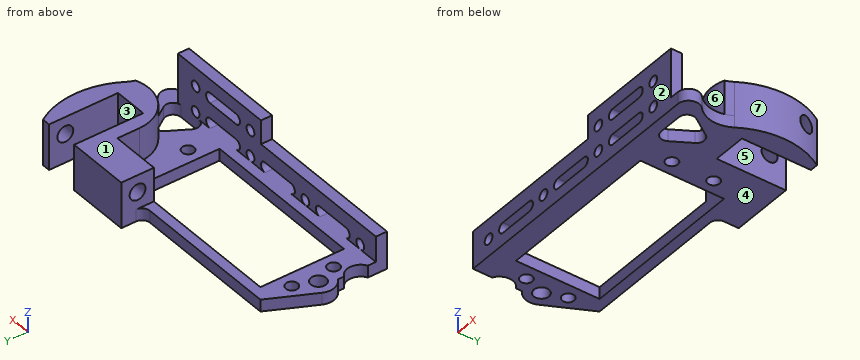
from build123d import *

# Parameters (mm, degrees)
SKETCH1_R           = 1.5
SKETCH1_R_2         = 1.9
SKETCH1_W           = 41.5
SKETCH1_H           = 21
BOSS_EXTRUDE1_DEPTH = 3
BOSS_EXTRUDE2_DEPTH = 8.5
BOSS_EXTRUDE3_DEPTH = 12.4
SKETCH4_R           = 1.3
CUT_EXTRUDE1_DEPTH  = 12.4
SKETCH5_W           = 38.3
SKETCH5_H           = 6
CUT_EXTRUDE2_DEPTH  = 12.4
SKETCH6_R           = 2
CUT_EXTRUDE3_DEPTH  = 42.4


with BuildPart() as part:
    # Sketch1 → Boss-Extrude1 (new body)
    with BuildSketch(Plane.XY):
        with BuildLine():
            Line((-3.321392505, 23.5), (33.5, 23.5))
            ThreePointArc((33.5, 23.5), (34.914213562, 24.085786438), (35.5, 25.5))
            Line((35.5, 25.5), (35.5, 29.2))
            Line((35.5, 29.2), (51.2, 29.2))
            Line((51.2, 29.2), (51.2, 11.85))
            Line((51.2, 11.85), (59.6, 11.85))
            Line((59.6, 11.85), (59.6, 29.2))
            Line((59.6, 29.2), (61.598774259, 29.2))
            ThreePointArc((61.598774259, 29.2), (64.6, 18.815792472), (61.598774259, 8.431584945))
            ThreePointArc((61.598774259, 8.431584945), (60.564280065, 3.6748318), (62.825022394, -0.636307591))
            ThreePointArc((62.825022394, -0.636307591), (63.518866569, -3.587010054), (61.018120639, -5.3))
            Line((61.018120639, -5.3), (-7.3, -5.3))
            Line((-7.3, -5.3), (-7.3, -0.5))
            ThreePointArc((-7.3, -0.5), (-5.5, 2.5), (-7.3, 5.5))
            Line((-7.3, 5.5), (-7.3, 7.067398479))
            ThreePointArc((-7.3, 7.067398479), (-9.16671437, 9.322502878), (-8.93851269, 12.241071429))
            Line((-8.93851269, 12.241071429), (-3.321392505, 23.5))
        make_face()
        with Locations((-3.5, 15.75)):
            Circle(SKETCH1_R, mode=Mode.SUBTRACT)
        with Locations((-5.448717527, 10.5)):
            Circle(SKETCH1_R_2, mode=Mode.SUBTRACT)
        with Locations((-3.5, 5.25)):
            Circle(SKETCH1_R, mode=Mode.SUBTRACT)
        with Locations((45, 5.25)):
            Circle(SKETCH1_R, mode=Mode.SUBTRACT)
        with Locations((45, 15.75)):
            Circle(SKETCH1_R, mode=Mode.SUBTRACT)
        with Locations((20.75, 10.5)):
            Rectangle(SKETCH1_W, SKETCH1_H, mode=Mode.SUBTRACT)
        with BuildLine():
            Line((49.961498231, 0.517681209), (52.768212791, 5.266104179))
            ThreePointArc((52.768212791, 5.266104179), (54.433574671, 6.247628711), (56.151588007, 5.361484945))
            Line((56.151588007, 5.361484945), (59.33232839, 0.613061975))
            ThreePointArc((59.33232839, 0.613061975), (59.435061822, -1.441773872), (57.670674684, -2.5))
            Line((57.670674684, -2.5), (51.683219741, -2.5))
            ThreePointArc((51.683219741, -2.5), (49.946072306, -1.491119968), (49.961498231, 0.517681209))
        make_face(mode=Mode.SUBTRACT)
    extrude(amount=BOSS_EXTRUDE1_DEPTH)

    # Sketch2 → Boss-Extrude2 (add)
    with BuildSketch(Plane.XY.offset(3)):
        with BuildLine():
            Line((61.598774259, 29.2), (59.6, 29.2))
            Line((59.6, 29.2), (59.6, 11.85))
            Line((59.6, 11.85), (51.2, 11.85))
            Line((51.2, 11.85), (51.2, 29.2))
            Line((51.2, 29.2), (35.5, 29.2))
            Line((35.5, 29.2), (35.5, 21))
            Line((35.5, 21), (47.7, 21))
            Line((47.7, 21), (47.7, 15.472440326))
            ThreePointArc((47.7, 15.472440326), (51.882998061, 7.567370729), (60.771830096, 6.579310435))
            ThreePointArc((60.771830096, 6.579310435), (61.119060066, 7.535021345), (61.598774259, 8.431584945))
            ThreePointArc((61.598774259, 8.431584945), (64.6, 18.815792472), (61.598774259, 29.2))
        make_face()
    extrude(amount=BOSS_EXTRUDE2_DEPTH)

    # Sketch3 → Boss-Extrude3 (add)
    with BuildSketch(Plane.XY.offset(3)):
        Polygon((46.39680607, -5.3), (-7.3, -5.3), (-7.3, -2.5), (58.7, -2.5), (58.7, -5.3), align=None)
    extrude(amount=BOSS_EXTRUDE3_DEPTH)

    # Sketch4 → Cut-Extrude1 (cut)
    with BuildSketch(Plane(origin=(0, -2.5, 0), x_dir=(1, 0, 0), z_dir=(0, 1, 0))):
        with Locations((52.8, -4.3)):
            Circle(SKETCH4_R)
        with Locations((34.5, -4.3)):
            Circle(SKETCH4_R)
        with Locations((52.8, -10.7)):
            Circle(SKETCH4_R)
        with Locations((34.5, -10.7)):
            Circle(SKETCH4_R)
        with Locations((16.2, -10.7)):
            Circle(SKETCH4_R)
        with Locations((-2.1, -10.7)):
            Circle(SKETCH4_R)
        with Locations((16.2, -4.3)):
            Circle(SKETCH4_R)
        with Locations((-2.1, -4.3)):
            Circle(SKETCH4_R)
        with BuildLine():
            Line((48, -5.6), (39.3, -5.6))
            ThreePointArc((39.3, -5.6), (38, -4.3), (39.3, -3))
            Line((39.3, -3), (48, -3))
            ThreePointArc((48, -3), (49.3, -4.3), (48, -5.6))
        make_face()
        with BuildLine():
            Line((48, -12), (39.3, -12))
            ThreePointArc((39.3, -12), (38, -10.7), (39.3, -9.4))
            Line((39.3, -9.4), (48, -9.4))
            ThreePointArc((48, -9.4), (49.3, -10.7), (48, -12))
        make_face()
        with BuildLine():
            Line((29.7, -12), (21, -12))
            ThreePointArc((21, -12), (19.7, -10.7), (21, -9.4))
            Line((21, -9.4), (29.7, -9.4))
            ThreePointArc((29.7, -9.4), (31, -10.7), (29.7, -12))
        make_face()
        with BuildLine():
            Line((11.4, -12), (2.7, -12))
            ThreePointArc((2.7, -12), (1.4, -10.7), (2.7, -9.4))
            Line((2.7, -9.4), (11.4, -9.4))
            ThreePointArc((11.4, -9.4), (12.7, -10.7), (11.4, -12))
        make_face()
        with BuildLine():
            Line((29.7, -5.6), (21, -5.6))
            ThreePointArc((21, -5.6), (19.7, -4.3), (21, -3))
            Line((21, -3), (29.7, -3))
            ThreePointArc((29.7, -3), (31, -4.3), (29.7, -5.6))
        make_face()
        with BuildLine():
            Line((11.4, -5.6), (2.7, -5.6))
            ThreePointArc((2.7, -5.6), (1.4, -4.3), (2.7, -3))
            Line((2.7, -3), (11.4, -3))
            ThreePointArc((11.4, -3), (12.7, -4.3), (11.4, -5.6))
        make_face()
    extrude(amount=-CUT_EXTRUDE1_DEPTH, mode=Mode.SUBTRACT)

    # Sketch5 → Cut-Extrude2 (cut)
    with BuildSketch(Plane(origin=(0, -2.5, 0), x_dir=(1, 0, 0), z_dir=(0, 1, 0))):
        with Locations((11.85, -12.4)):
            Rectangle(SKETCH5_W, SKETCH5_H)
    extrude(amount=-CUT_EXTRUDE2_DEPTH, mode=Mode.SUBTRACT)

    # Sketch6 → Cut-Extrude3 (cut)
    with BuildSketch(Plane.ZY.offset(-35.5)):
        with Locations((7.25, 25.1)):
            Circle(SKETCH6_R)
    extrude(amount=-CUT_EXTRUDE3_DEPTH, mode=Mode.SUBTRACT)


solid = part.part
Design review of the part built by this model. Coordinates are the model's own, in mm. Face numbers are marked on the shaded views. A direction names the side the tool comes from. Coordinates: 2 decimals unless noted, no trailing zeros. Write each loop counter-clockwise with the first axis right and the second up, starting at its lowest first coordinate (ties: lowest second). Pieces come first, ordered by that corner, then holes. Notation, with made-up numbers: (75.25, 66) -> (130.25, 66) arc R28 cw to (130.25, 85) -> close; hole circle Ø2 at (15, 39). An arc over 180 degrees is marked (long way). Write each question's results on one line, items separated by ' | '. Start each with the question number.
(1) For line 1 along Y through (x, z) = (45, 2); line 2 along X through (y, z) = (-3.65, 10.7); line 3 along Y through (x, z) = (7, 1), list the stretches that pass through material, from the lowest coordinate up. Write a range as from..to.
(2) The part is to be moulded in two halves that separate along X. For the marked faces 4, 5, 6 and 7, say which applies: pulls with the +X half, pulls with the -X half, needs draft (parallel to the pull), parting line crosses it, or undercut.
(3) Take a section at A-A on x = 29. Write out the cut boundary in (y, z).
(4) Clearance check with flat-ended pins moving along their axes: P1, Ø2.5, axis at y = -2, z = 5.5, coming from the -X side; P2, Ø3, axis at x = 45, y = -4.5, coming from the -Z side; P3, Ø3.5, axis at y = 11, z = 2, coming from the +X side; P4, Ø8, axis at y = 20.5, z = 2.5, coming from the -X side. State where each tip first meets the part, or that it passes through.
(5) Tool access review of the marked faces 1, 2 and 3: name each direction out of +Z, -Z, +X, -X, +Y, -Y from which nothing blocks a thin tool from reaching the whole face with its end or side.
(6) Take a section at B-B on z = 4.3. Give the number of separate pieces and of enclosed holes in the cut face, and give its area (3 significant figures).
Results found:
1) line 1: y = -5.3..3.75, 6.75..14.25, 17.25..29.2 | line 2: x = 31..33.2, 35.8..38, 49.3..51.5, 54.1..58.7 | line 3: y = -5.3..0, 21..23.5
2) face 4: needs draft | face 5: undercut | face 6: parting line crosses it | face 7: pulls with the +X half
3) outline: (-5.3, 0) -> (0, 0) -> (0, 3) -> (-5.3, 3) -> close; (-5.3, 5.6) -> (-2.5, 5.6) -> (-2.5, 9.4) -> (-5.3, 9.4) -> close; (21, 0) -> (23.5, 0) -> (23.5, 3) -> (21, 3) -> close
4) P1: stops at x = -7.3 | P2: stops at z = 0 | P3: stops at x = 63.63 | P4: stops at x = -6.81
5) face 1: +Z, +X, -X, +Y | face 2: +Z, -Z, +X, -X, -Y | face 3: +Z, -Z, +Y
6) separate pieces: 9 | enclosed holes: 0 | area: 359 mm2
